from build123d import *

# Parameters (mm, degrees)
F0_W      = 101.6
F0_H      = 101.6
F1_DEPTH  = 7
F3_DEPTH  = 6
F4_W      = 5
F4_H      = 57.6000098
F5_DEPTH  = 6
F6_W      = 6
F6_H      = 29.5999916
F6_W_2    = 4
F6_W_3    = 4.6
F6_H_2    = 21.5999916
F7_DEPTH  = 6
F9_DEPTH  = 6
F11_DEPTH = 6
F12_W     = 22.6
F12_H     = 1
F13_DEPTH = 6
F15_DEPTH = 6


with BuildPart() as f1:
    # F0 (on Top) → F1 (new body)
    with BuildSketch(Plane.XY):
        Rectangle(F0_W, F0_H)
    extrude(amount=F1_DEPTH)

    # F2 (on face) → F3 (cut)
    with BuildSketch(Plane.XY.offset(7)):
        Polygon((-1.2, -42.8), (-1.2, -41.8), (19.8, -41.8), (19.8, -28.8), (-1.2, -28.8), (-1.2, -27.8), (19.8, -27.8), (19.8, -21.8), (-7.2, -21.8), (-7.2, -34.8), (13.8, -34.8), (13.8, -35.8), (-7.2, -35.8), (-7.2, -48.8), (50.8, -48.8), (50.8, -42.8), align=None)
    extrude(amount=-F3_DEPTH, mode=Mode.SUBTRACT)

    # F4 (on face) → F5 (cut)
    with BuildSketch(Plane.XY.offset(7)):
        with Locations((-48.3, 21.9999951)):
            Rectangle(F4_W, F4_H)
        Polygon((-44.8, 50.8), (-44.8, -6.8000098), (-30.8, -6.8000098), (-30.8, 50.8), (-37.8, 50.8), (-37.8, -0.8000098), (-38.8, -0.8000098), (-38.8, 50.8), align=None)
    extrude(amount=-F5_DEPTH, mode=Mode.SUBTRACT)

    # F6 (on face) → F7 (cut)
    with BuildSketch(Plane.XY.offset(7)):
        with Locations((-26.8, 36.0000042)):
            Rectangle(F6_W, F6_H)
        with Locations((-20.8, 36.0000042)):
            Rectangle(F6_W_2, F6_H)
        Polygon((-17.8, 50.8), (-17.8, 21.2000084), (0.8, 21.2000084), (0.8, 43.8), (1.8, 43.8), (1.8, 21.2000084), (14.8, 21.2000084), (14.8, 43.8), (15.8, 43.8), (15.8, 21.2000084), (28.8, 21.2000084), (28.8, 43.8), (29.8, 43.8), (29.8, 21.2000084), (42.8, 21.2000084), (42.8, 43.8), (43.8, 43.8), (43.8, 21.2000084), (49.8, 21.2000084), (49.8, 49.8), (36.8, 49.8), (36.8, 27.2000084), (35.8, 27.2000084), (35.8, 49.8), (22.8, 49.8), (22.8, 27.2000084), (21.8, 27.2000084), (21.8, 49.8), (8.8, 49.8), (8.8, 27.2000084), (7.8, 27.2000084), (7.8, 49.8), (-5.2, 49.8), (-5.2, 28.2000084), (-5.2, 27.2000084), (-6.2, 27.2000084), (-10.8, 27.2000084), (-11.8, 27.2000084), (-11.8, 28.2000084), (-11.8, 49.8), (-11.8, 50.8), align=None)
        with Locations((-8.5, 39.0000042)):
            Rectangle(F6_W_3, F6_H_2)
    extrude(amount=-F7_DEPTH, mode=Mode.SUBTRACT)

    # F8 (on face) → F9 (cut)
    with BuildSketch(Plane.XY.offset(7)):
        Polygon((-29.8, 21.2000084), (-29.8, 14.2000084), (-1.8, 14.2000084), (-1.8, -13.8), (19.8, -13.8), (20.8, -13.8), (20.8, -41.8), (50.8, -41.8), (50.8, -35.8), (26.8, -35.8), (26.8, -34.8), (26.8, -6.8), (4.2, -6.8), (4.2, 20.2000084), (-22.8, 20.2000084), (-23.8, 20.2000084), (-23.8, 21.2000084), align=None)
    extrude(amount=-F9_DEPTH, mode=Mode.SUBTRACT)

    # F10 (on face) → F11 (cut)
    with BuildSketch(Plane.XY.offset(7)):
        Polygon((49.8, 21.2000084), (43.8, 21.2000084), (43.8, 20.2000084), (5.2, 20.2000084), (5.2, 7.2000084), (43.8, 7.2000084), (43.8, 6.2000084), (5.2, 6.2000084), (5.2, -5.8), (5.2, -6.8), (26.8, -6.8), (43.8, -6.8), (43.8, -7.8), (34.8, -7.8), (34.8, -13.8), (43.8, -13.8), (43.8, -14.8), (34.8, -14.8), (34.8, -27.8), (43.8, -27.8), (43.8, -28.8), (34.8, -28.8), (33.8, -28.8), (33.8, -7.8), (26.8, -7.8), (26.8, -13.8), (27.8, -13.8), (27.8, -34.8), (49.8, -34.8), (49.8, -21.8), (40.8, -21.8), (40.8, -20.8), (49.8, -20.8), (49.8, -7.8), (49.8, -6.8), (49.8, -0.7999916), (11.2, -0.7999916), (11.2, 0.2000084), (49.8, 0.2000084), (49.8, 13.2000084), (11.2, 13.2000084), (11.2, 14.2000084), (49.8, 14.2000084), align=None)
    extrude(amount=-F11_DEPTH, mode=Mode.SUBTRACT)

    # F12 (on face) → F13 (join)
    with BuildSketch(Plane.XY.offset(1)):
        with Locations((15.5, -7.3)):
            Rectangle(F12_W, F12_H)
    extrude(amount=F13_DEPTH)

    # F14 (on face) → F15 (cut)
    with BuildSketch(Plane.XY.offset(7)):
        Polygon((-29.8, -6.8000098), (-29.8, -7.8000098), (-49.8, -7.8000098), (-49.8, -20.8000098), (-22.8, -20.8000098), (-22.8, -21.8), (-42.2, -21.8), (-42.2, -27.8), (-42.2, -50.8), (-36.2, -50.8), (-36.2, -27.8), (-35.2, -27.8), (-35.2, -50.8), (-29.2, -50.8), (-29.2, -27.8), (-28.2, -27.8), (-28.2, -50.8), (-22.2, -50.8), (-22.2, -27.8), (-21.2, -27.8), (-21.2, -50.8), (-15.2, -50.8), (-15.2, -27.8), (-14.2, -27.8), (-14.2, -50.8), (-8.2, -50.8), (-8.2, -21.8), (-16.8, -21.8), (-16.8, -20.8000098), (-16.8, -14.8000098), (-43.8, -14.8000098), (-43.8, -13.8000098), (-16.8, -13.8000098), (-16.8, 7.2000084), (-15.8, 7.2000084), (-8.8, 7.2000084), (-8.8, 6.2000084), (-15.8, 6.2000084), (-15.8, -6.7999916), (-8.8, -6.7999916), (-8.8, -7.7999916), (-15.8, -7.7999916), (-15.8, -14.8000098), (-15.8, -20.8000098), (19.8, -20.8000098), (19.8, -14.8), (-2.8, -14.8), (-9.8, -14.8), (-9.8, -13.8), (-2.8, -13.8), (-2.8, -0.7999916), (-9.8, -0.7999916), (-9.8, 0.2000084), (-2.8, 0.2000084), (-2.8, 13.2000084), (-22.8, 13.2000084), (-22.8, -7.8000098), (-23.8, -7.8000098), (-23.8, 14.2000084), (-29.8, 14.2000084), align=None)
        Polygon((-43.2, -21.8), (-50.8, -21.8), (-50.8, -50.8), (-43.2, -50.8), (-43.2, -27.8), align=None)
    extrude(amount=-F15_DEPTH, mode=Mode.SUBTRACT)


solid = f1.part
For this review, take the finished solid that the model builds, in its own axes (mm). A direction names the side the tool comes from. Round coordinates to 2 decimals unless told otherwise and drop trailing zeros. One line per item, written item: value. Start each with the question number.
Item 1: Take a section at A-A (z = 3.5). State how many separate pieces and enclosed holes the cut face has, plus the area to 3 significant figures.
Item 2: For L1, parallel to X at y = -23, z = 3; L2, parallel to Y at x = -12, z = 6; L3, parallel to X at y = -45.5, z = 5, list the stretches that pass through material, from the lowest coordinate up.
Item 3: Clearance check with flat-ended pins moving along their axes: pin 1 Ø6 at (x, y) = (30, 5) entering from -Z; pin 2 Ø1.8 at (y, z) = (19, 4) entering from -X; pin 3 Ø1.2 at (x, y) = (-21.5, 33.5) entering from +Z; pin 4 Ø0.5 at (x, z) = (-21.5, 5.5) entering from +Y. State where each tip first meets the part, or that it passes through.
Item 4: The part is to be moulded in two halves that separate along X. For faces 1 (the flat face through (50.8, -1, 3)), 2 (the flat face through (-47, -21.8, 4)), 3 (the flat face through (-30, -14.8, 4)), say which applies: +X half, -X half, draft (parallel to the pull), parting line (faces both ways), or undercut.
Item 5: For faces 4 (the flat face through (-44.8, 22, 4)), 5 (the flat face through (22.8, 39, 4)), 6 (the flat face through (-45, 4, 7)), 7 (the flat face through (-14.2, -39, 4)), list the 3-axis set-ups (+Z, -Z, +X, -X, +Y, -Y) from which the entire face can be reached by the end or side of a thin tool; tool diameter is ignored.
Answer below:
1. separate pieces: 9
1. enclosed holes: 1
1. area: 1,590 mm2
2. L1: x = -43.2 to -42.2, -8.2 to -7.2, 19.8 to 20.8, 26.8 to 27.8, 33.8 to 34.8, 49.8 to 50.8
2. L2: y = -21.8 to -20.8, -7.8 to -6.8, 6.2 to 7.2, 13.2 to 14.2, 20.2 to 21.2
2. L3: x = -43.2 to -42.2, -36.2 to -35.2, -29.2 to -28.2, -22.2 to -21.2, -15.2 to -14.2, -8.2 to -7.2
3. pin 1: stops at z = 0
3. pin 2: stops at x = -45.8
3. pin 3: stops at z = 1
3. pin 4: stops at y = 21.2
4. face 1: +X half
4. face 2: draft
4. face 3: undercut
5. face 4: +Z, +Y
5. face 5: +Z
5. face 6: +Z, +X, -X, +Y, -Y
5. face 7: +Z, -Y
